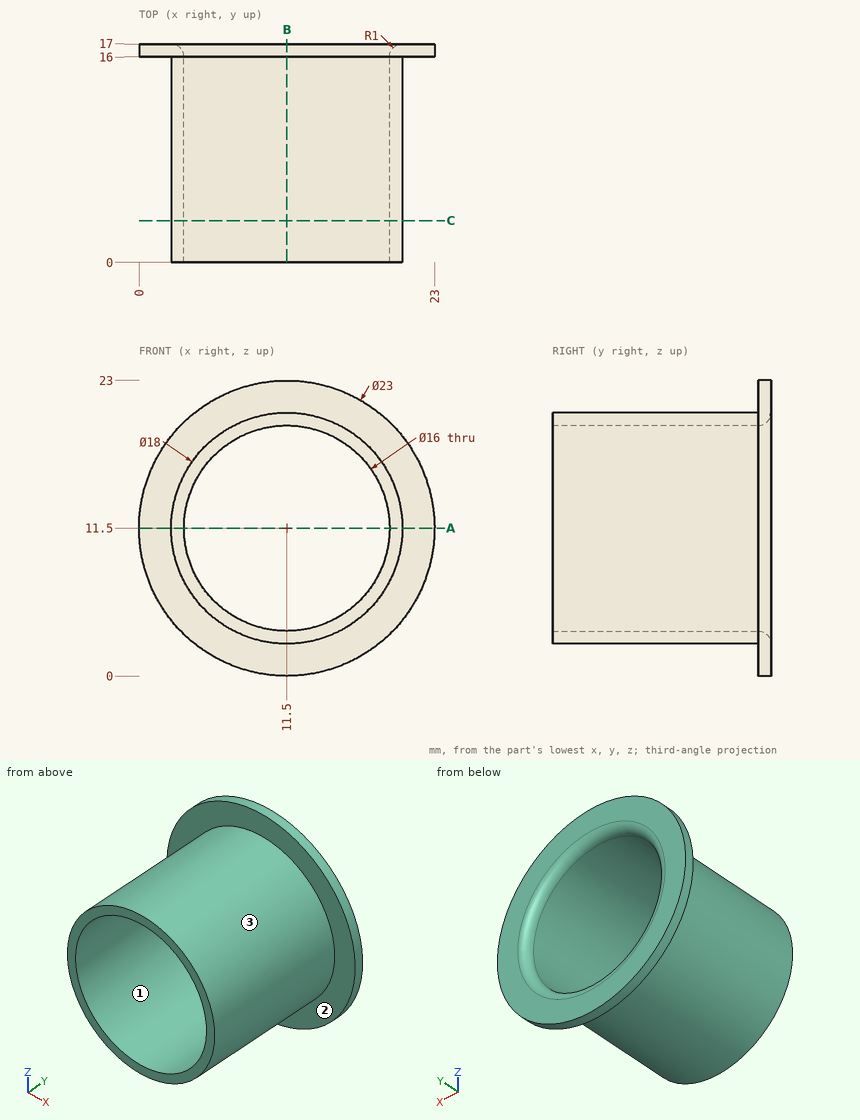
Could you check a few things on this drawing? It's one solid part, dimensions in mm from its lowest x, y, z. Coordinates: 2 decimals unless noted, no trailing zeros. Order: outer loops, then holes, each group sorted by start corner. A loop starts at its lowest first (then second) coordinate and runs counter-clockwise, first axis right, second up. Notation, with made-up numbers: (53, -12) - (88, -12) arc R32 cw to (88, 16) - close; hole circle Ø3 at (80, 7.5). An arc over 180 degrees is marked (long way). Answer as a JSON object with one key per item and string values. Group by question number.
Q1. Imagine slicing it at B-B (x = 11.5). Please give me the cut outline in (y, z), and give its area (3 significant figures).
Q2. Imagine slicing it at A-A (z = 11.5). Please give me the cut outline in (x, y), and give its area (3 significant figures).
Q3. Will these pins go through, and if not, where does the flat tip stop? P1, Ø3, axis at x = 3.5, z = 3.5, coming from the -Y side; P2, Ø6, axis at x = 5, y = 10.5, coming from the -Z side; P3, Ø4, axis at x = 19.5, y = 13.5, coming from the -Z side.
Q4. Imagine slicing it at C-C (y = 3.25). Please give me the cut outline in (x, z), and give its area (3 significant figures).
Q5. I need wall thicknesses on line 1 (X direction, y = 7.75, z = 11.25); line 2 (Y direction, x = 21.5, z = 7.75). Which ranges of each line are inside material? Lowest first, please. Write a range as from..to.
Q6. We'd pull the mould along X, two halves only. Please class the marked faces 1, 2 and 3: +X half, -X half, draft (parallel to the pull), parting line (faces both ways), or undercut.
Determined:
{
 "1": {"outline": "(0, 2.5) - (16, 2.5) - (16, 0) - (17, 0) - (17, 2.5) arc R1 ccw to (16, 3.5) - (0, 3.5) - close; (0, 19.5) - (16, 19.5) arc R1 ccw to (17, 20.5) - (17, 23) - (16, 23) - (16, 20.5) - (0, 20.5) - close", "area": "38.6 mm2"},
 "2": {"outline": "(0, 16) - (2.5, 16) - (2.5, 0) - (3.5, 0) - (3.5, 16) arc R1 ccw to (2.5, 17) - (0, 17) - close; (19.5, 0) - (20.5, 0) - (20.5, 16) - (23, 16) - (23, 17) - (20.5, 17) arc R1 ccw to (19.5, 16) - close", "area": "38.6 mm2"},
 "3": {"P1": "stops at y = 16", "P2": "stops at z = 3.21", "P3": "stops at z = 4.79"},
 "4": {"outline": "circle Ø18 at (11.5, 11.5); hole circle Ø16 at (11.5, 11.5)", "area": "53.4 mm2"},
 "5": {"line 1": "x = 2.5..3.5, 19.5..20.5", "line 2": "y = 16..17"},
 "6": {"face 1": "undercut", "face 2": "draft", "face 3": "parting line"}
}
